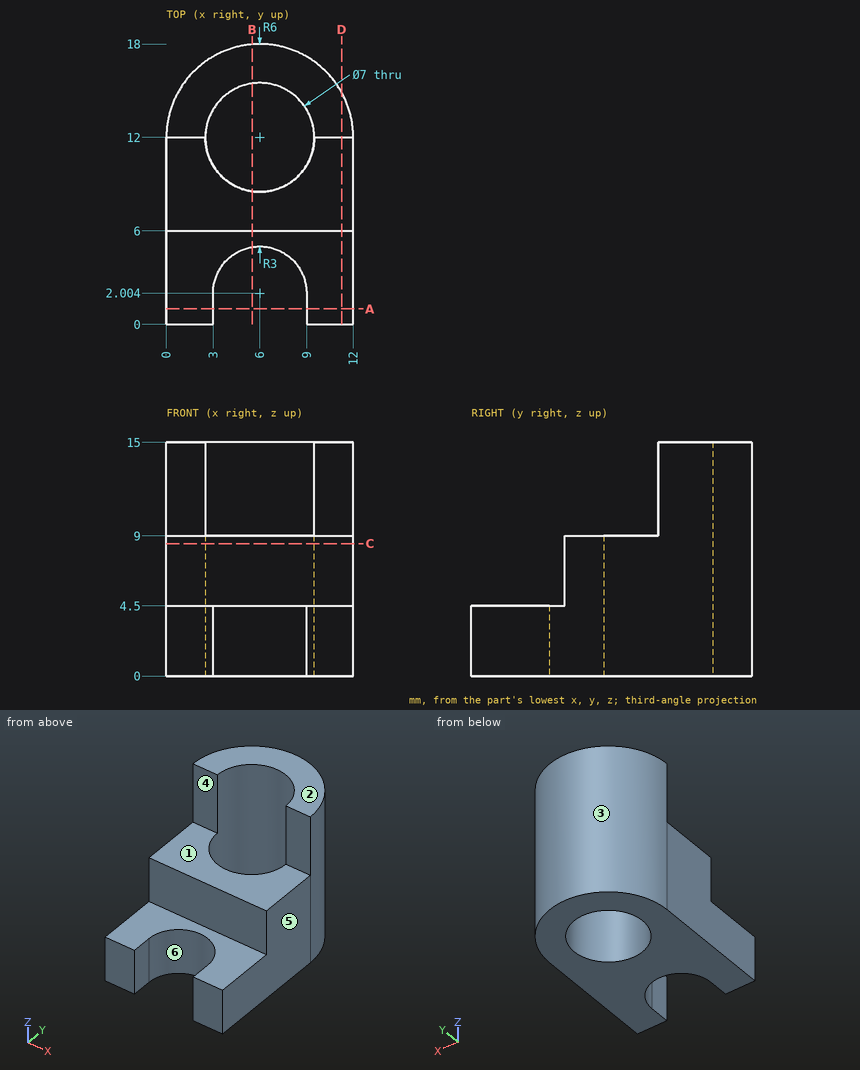
The figure shows three views and two pictorial views of one solid part (mm, origin at its lowest corner). Answer the questions. A direction names the side the tool comes from. Give positions to 0.01 mm unless a question says otherwise; leave off trailing zeros. Write each loop counter-clockwise with the first axis right and the second up, starting at its lowest first coordinate (ties: lowest second). Pieces come first, ordered by that corner, then holes. Notation, with made-up numbers: (49, 45) - (54, 45) arc R31 cw to (54, 77) - close; hole circle Ø11 at (66.5, -22.5). An arc over 180 degrees is marked (long way). Use CSV: the item, a comma, the result in double quotes. Start each with the question number.
Item 1: For the marked faces 1 and 2, determine the directions among +Z, -Z, +X, -X, +Y, -Y from which every point of the face is accessible in a straight line to the end or side of a thin tool.
Item 2: The part is cut by section B-B, the plane x = 5.5. Give the vertices of the cut face in (y, z).
Item 3: Consider line 1 (X direction, y = 12, z = 8.75); line 2 (Y direction, x = 6, z = 7.25); line 3 (X direction, y = 1.25, z = 1.5). Determine where each line is inside the solid, lowest interval first.
Item 4: The part is cut by section A-A, the plane y = 1. Give the vertices of the cut face in (x, z).
Item 5: Flat-ended cylindrical pins translate along their axes: P1, Ø3, axis at x = 11, z = 12.5, coming from the -Y side; P2, Ø3, axis at x = 1.5, y = 14, coming from the -Z side; P3, Ø1.8, axis at x = 7.5, y = 3, coming from the +Z side; P4, Ø6, axis at x = 1.5, z = 5, coming from the +Y side. Find the tip coordinate at first contact, or state that the pin passes through.
Item 6: The mould has two halves that part along X. Classify the marked faces 3, 4, 5 and 6: pulls with the +X half, pulls with the -X half, needs draft (parallel to the pull), parting line crosses it, or undercut.
Item 7: The part is cut by section C-C, the plane z = 8.5. Give the vertices of the cut face in (x, y).
Item 8: The part is cut by section D-D, the plane x = 11.25. Give the vertices of the cut face in (y, z) (1 decimal).
Taken from the geometry:
1,face 1,"+Z, +X, -X, -Y"
1,face 2,"+Z, +X, -X, +Y, -Y"
2,outline,"(4.96, 0) - (8.54, 0) - (8.54, 9) - (6, 9) - (6, 4.5) - (4.96, 4.5) - close; (15.46, 0) - (17.98, 0) - (17.98, 15) - (15.46, 15) - close"
3,line 1,"0 to 2.5, 9.5 to 12"
3,line 2,"6 to 8.5, 15.5 to 18"
3,line 3,"0 to 3, 9 to 12"
4,outline,"(0, 0) - (3, 0) - (3, 4.5) - (0, 4.5) - close; (9, 0) - (12, 0) - (12, 4.5) - (9, 4.5) - close"
5,P1,"y = 12"
5,P2,"z = 0"
5,P3,"through"
5,P4,"y = 17.81"
6,face 3,"parting line crosses it"
6,face 4,"needs draft"
6,face 5,"pulls with the +X half"
6,face 6,"undercut"
7,outline,"(0, 6) - (12, 6) - (12, 12) arc R6 ccw to (0, 12) - close; hole circle Ø7 at (6, 12)"
8,outline,"(0, 0) - (14.9, 0) - (14.9, 15) - (12, 15) - (12, 9) - (6, 9) - (6, 4.5) - (0, 4.5) - close"
